Geometry check sheet. Reference: the model listing, model coordinates, mm. A direction names the side the tool comes from. Round coordinates to 2 decimals unless told otherwise and drop trailing zeros. Write each loop counter-clockwise with the first axis right and the second up, starting at its lowest first coordinate (ties: lowest second). Pieces come first, ordered by that corner, then holes. Notation, with made-up numbers: (87.5, -17) - (131.5, -17) arc R22 cw to (131.5, -2) - close; hole circle Ø4 at (-37.75, -3). An arc over 180 degrees is marked (long way). Return JSON: item names as keys, results as strings. Group by question number.
from build123d import *

# Parameters (mm, degrees)
BOSS_EXTRUDE1_DEPTH = 63.5
SKETCH3_W           = 781.722843432
SKETCH3_H           = 58.42
BOSS_EXTRUDE2_DEPTH = 152.4


with BuildPart() as part:
    # Sketch2 → Boss-Extrude1 (new body)
    with BuildSketch(Plane.XY):
        with BuildLine():
            Line((390.861421716, -251.565063977), (390.861421716, -984.152448319))
            Line((390.861421716, -984.152448319), (-390.861421716, -984.152448319))
            Line((-390.861421716, -984.152448319), (-390.861421716, -251.565063977))
            ThreePointArc((-390.861421716, -251.565063977), (0, -464.82), (390.861421716, -251.565063977))
        make_face()
    extrude(amount=BOSS_EXTRUDE1_DEPTH)

    # Sketch3 → Boss-Extrude2 (add)
    with BuildSketch(Plane.XY.offset(63.5)):
        with Locations((0, -954.942448319)):
            Rectangle(SKETCH3_W, SKETCH3_H)
    extrude(amount=BOSS_EXTRUDE2_DEPTH)


solid = part.part
1. Section check C-C (z = 158.5). Enter the section's corners in (x, y), and give its area (3 significant figures).
2. Tool access check on faces 4 (the face through (5, -659, 63.5)), 5 (the face through (-5, -984.152, 106)). Record the directions out of +Z, -Z, +X, -X, +Y, -Y that give a thin tool (end or side, any length) a straight path to the whole face; none if there is none.
3. Material ranges on line 1 along Y through (x, z) = (-33, 167); line 2 along Z through (x, y) = (158.5, -790.5); line 3 along X through (y, z) = (-388, 62), recorded low to high.
4. Section check D-D (y = -861.5). Enter the section's corners in (x, z).
5. Depth check by flat-ended pin: pin 1 Ø4 at (x, z) = (198, 128) entering from +Y; pin 2 Ø4 at (x, y) = (43, -812) entering from -Z; pin 3 Ø5 at (x, y) = (-224, -633.5) entering from +Z; pin 4 Ø1.5 at (x, z) = (165.5, 45) entering from +Y. Enter the tip coordinate at first touch or a pass-through.
6. Section check B-B (x = 323.5). Enter the section's corners in (y, z), and give its area (3 significant figures).
7. Mould release check, pull along X, two halves, no side actions. Record for faces 1 (the face through (-390.861, -704, 58)), 2 (the face through (-6.5, -464.775, 31.306)), 3 (the face through (-5, -925.732, 139)): pulls with the +X half, pulls with the -X half, needs draft (parallel to the pull), parting line crosses it, or undercut.
8. Section check A-A (y = -352.5). Enter the section's corners in (x, z), and give its area (3 significant figures).
Result sheet:
{
 "1": {"outline": "(-390.86, -984.15) - (390.86, -984.15) - (390.86, -925.73) - (-390.86, -925.73) - close", "area": "45,700 mm²"},
 "2": {"face 4": "+Z, +X, -X, +Y", "face 5": "+Z, -Z, +X, -X, -Y"},
 "3": {"line 1": "y = -984.15 to -925.73", "line 2": "z = 0 to 63.5", "line 3": "x = -390.86 to -255.96, 255.96 to 390.86"},
 "4": {"outline": "(-390.86, 0) - (390.86, 0) - (390.86, 63.5) - (-390.86, 63.5) - close"},
 "5": {"pin 1": "stops at y = -925.73", "pin 2": "stops at z = 0", "pin 3": "stops at z = 63.5", "pin 4": "stops at y = -434.07"},
 "6": {"outline": "(-984.15, 0) - (-333.77, 0) - (-333.77, 63.5) - (-925.73, 63.5) - (-925.73, 215.9) - (-984.15, 215.9) - close", "area": "50,200 mm²"},
 "7": {"face 1": "pulls with the -X half", "face 2": "undercut", "face 3": "needs draft"},
 "8": {"outline": "(-390.86, 0) - (-302.99, 0) - (-302.99, 63.5) - (-390.86, 63.5) - close; (302.99, 0) - (390.86, 0) - (390.86, 63.5) - (302.99, 63.5) - close", "area": "11,200 mm²"}
}
